Geometry: see drawing. Coordinates: mm, zero at the bounding-box minimum. Coordinates: 2 decimals unless noted, no trailing zeros. Loops run counter-clockwise (first coordinate to the right, second up) from the corner with the lowest first, then second, coordinate; pieces in that order, holes last. Notation, with made-up numbers: (74, -39) - (87, -39) arc R30 cw to (87, -5) - close; hole circle Ø5 at (33, 85.25). An arc over 180 degrees is marked (long way). Use a Markdown table: item, result. Add a question column.
1. Section query A-A on y = 10. Return the cut outline in (x, z), then the cut area to 3 significant figures.
2. Ray query, L1, parallel to Z at x = 7.25, y = 10; L2, parallel to Y at x = 4, z = 10.75; L3, parallel to Z at x = 18.4, y = 50. Return the intervals inside material, ascending. Write a range as [from, to].
3. Section query D-D on y = 50. Return the cut outline in (x, z), then the cut area to 3 significant figures.
4. Section query B-B on z = 10. Return the cut outline in (x, y).
5. Section query C-C on x = 12.5. Return the cut outline in (y, z), then the cut area to 3 significant figures.
6. Contact query for a flat-ended pin moving along its axis: P1, Ø7, axis at y = 72.5, z = 10, coming from the +X side. Output: stop coordinate, or through.
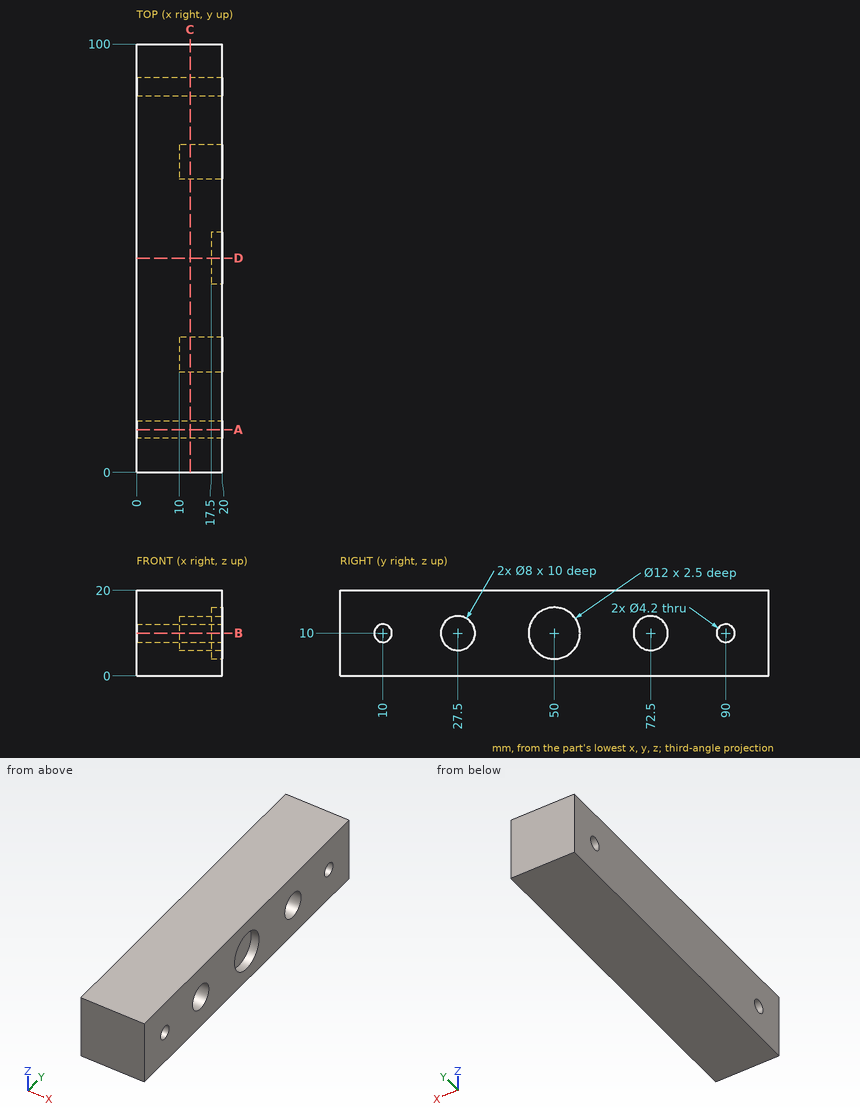
Resolved:
| question | item | result |
|---|---|---|
| 1 | outline | (0, 0) - (20, 0) - (20, 7.9) - (0, 7.9) - close; (0, 12.1) - (20, 12.1) - (20, 20) - (0, 20) - close |
| 1 | area | 316 mm² |
| 2 | L1 | [0, 7.9], [12.1, 20] |
| 2 | L2 | [0, 8.04], [11.96, 88.04], [91.96, 100] |
| 2 | L3 | [0, 4], [16, 20] |
| 3 | outline | (0, 0) - (20, 0) - (20, 4) - (17.5, 4) - (17.5, 16) - (20, 16) - (20, 20) - (0, 20) - close |
| 3 | area | 370 mm² |
| 4 | outline | (0, 0) - (20, 0) - (20, 7.9) - (0, 7.9) - close; (0, 12.1) - (20, 12.1) - (20, 23.5) - (10, 23.5) - (10, 31.5) - (20, 31.5) - (20, 44) - (17.5, 44) - (17.5, 56) - (20, 56) - (20, 68.5) - (10, 68.5) - (10, 76.5) - (20, 76.5) - (20, 87.9) - (0, 87.9) - close; (0, 92.1) - (20, 92.1) - (20, 100) - (0, 100) - close |
| 5 | outline | (0, 0) - (100, 0) - (100, 20) - (0, 20) - close; hole circle Ø4.2 at (10, 10); hole circle Ø8 at (27.5, 10); hole circle Ø8 at (72.5, 10); hole circle Ø4.2 at (90, 10) |
| 5 | area | 1,870 mm² |
| 6 | P1 | x = 10 |
